Input: dimensioned drawing with shaded views. Units: mm. Origin: part minimum x, y, z. A direction names the side the tool comes from. Round coordinates to 2 decimals unless told otherwise and drop trailing zeros. Write each loop counter-clockwise with the first axis right and the second up, starting at its lowest first coordinate (ties: lowest second). Pieces come first, ordered by that corner, then holes. Notation, with made-up numbers: M 10.5,0 L 55.5,0 A17 ccw 55.5,14 Z; hole C 38,86.25 d1. An arc over 180 degrees is marked long. Answer as CSV lines item,"result". Start each with the question number.
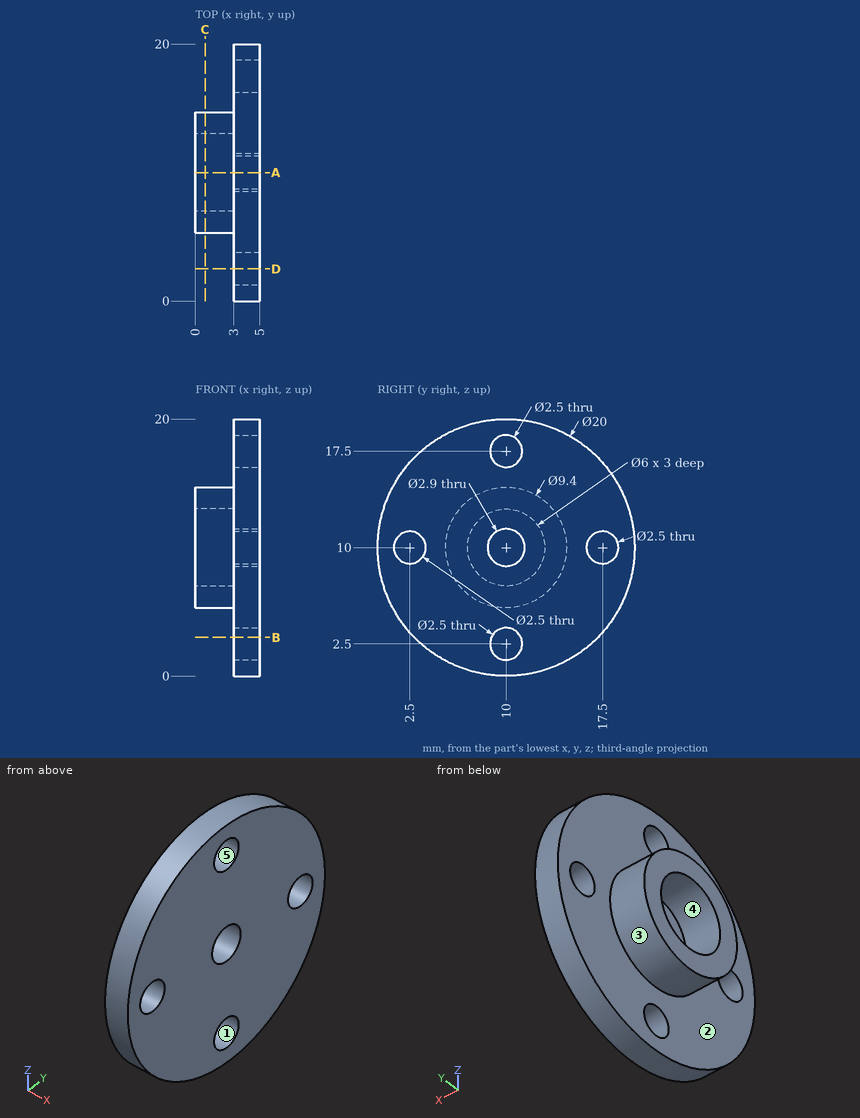
Item 1: Access query for the marked faces 4 and 5. Directions: +Z, -Z, +X, -X, +Y, -Y. A direction counts if a zero-diameter tool reaches every point of the face in a straight line with its end or side. Return the directions, or none.
Item 2: Cut plane B-B, the plane z = 3. Return loops of the section in (x, y), plus the area to 3 significant figures.
Item 3: Cut plane A-A, the plane y = 10. Return loops of the section in (x, z), plus the area to 3 significant figures.
Item 4: Cut plane D-D, the plane y = 2.5. Return loops of the section in (x, z).
Item 5: Line query: line 1 (Z direction, x = 3.8, y = 10); line 2 (Y direction, x = 1.7, z = 10); line 3 (X direction, y = 17, z = 5). Output: solid intervals per line, ascending. Write a range as [from, to].
Item 6: Pin query (flat end, axial travel): pin 1 Ø1 at (x, y) = (4, 3) entering from +Z; pin 2 Ø4 at (y, z) = (10, 17.5) entering from -X. Return the tip coordinate at first contact, or that it passes through.
Item 7: Cut plane C-C, the plane x = 0.75. Return loops of the section in (y, z).
Item 8: Draft query along Z for the marked faces 1, 2 and 3. Return one class per face: +Z half, -Z half, draft (parallel to the pull), parting line (faces both ways), or undercut.
Results list:
1,face 4,"-X"
1,face 5,"+X, -X"
2,outline,"M 3,2.86 L 5,2.86 L 5,8.85 L 3,8.85 Z; M 3,11.15 L 5,11.15 L 5,17.14 L 3,17.14 Z"
2,area,"24.0 mm²"
3,outline,"M 0,5.3 L 3,5.3 L 3,3.75 L 5,3.75 L 5,8.55 L 3,8.55 L 3,7 L 0,7 Z; M 0,13 L 3,13 L 3,11.45 L 5,11.45 L 5,16.25 L 3,16.25 L 3,14.7 L 0,14.7 Z; M 3,0 L 5,0 L 5,1.25 L 3,1.25 Z; M 3,18.75 L 5,18.75 L 5,20 L 3,20 Z"
3,area,"34.4 mm²"
4,outline,"M 3,3.39 L 5,3.39 L 5,8.75 L 3,8.75 Z; M 3,11.25 L 5,11.25 L 5,16.61 L 3,16.61 Z"
5,line 1,"[0, 1.25], [3.75, 8.55], [11.45, 16.25], [18.75, 20]"
5,line 2,"[5.3, 7], [13, 14.7]"
5,line 3,"[3, 5]"
6,pin 1,"z = 17.6"
6,pin 2,"x = 3"
7,outline,"C 10,10 d9.4; hole C 10,10 d6"
8,face 1,"undercut"
8,face 2,"draft"
8,face 3,"parting line"
